Work out the finished part from the listing and answer in its coordinate system (mm). A direction names the side the tool comes from. Coordinates: 2 decimals unless noted, no trailing zeros. Write each loop counter-clockwise with the first axis right and the second up, starting at its lowest first coordinate (ties: lowest second). Pieces come first, ordered by that corner, then holes. Notation, with made-up numbers: (48.25, 21) - (106.25, 21) arc R21 ccw to (106.25, 48) - close; hole circle Ø4 at (-22, -15). An arc over 180 degrees is marked (long way). Use one line per item in the form item = value. Start each with the question number.
Item 1: Given pin 1 (4.5 mm diameter, centred on x = -11.5, z = 3.5, fed in from -Y); pin 2 (2.5 mm diameter, centred on y = 9, z = 4, fed in from +X); pin 3 (4.5 mm diameter, centred on x = -14.5, z = 2.5, fed in from +Y), each flat-ended and moving along its own axis, determine where each tip first touches the part or whether it passes through.
Item 2: A cutting plane is placed at C-C (y = 24.5). Write down the section's boundary in (x, z).
Item 3: A cutting plane is placed at B-B (z = 4.5). Write down the section's boundary in (x, y).
Item 4: Consider probe 1 along Y at (x, z) = (-14.5, 8); probe 2 along X at (y, z) = (24.75, 8.75); probe 3 along Y at (x, z) = (-24, 0.5). Determine where each line is inside the solid, lowest interval first.
Item 5: A cutting plane is placed at A-A (x = -13.25). Write down the section's boundary in (y, z).
Item 6: Determine the mould class of faces 1 (the cylindrical face through (-25.568, 29.715, 9.699)), 2 (the flat face through (-13, 15, 1)), 3 (the cylindrical face through (-19.606, 1.426, 5.056)) for opening direction Y: released by +Y, released by -Y, zero draft, split by the parting line, or undercut.
Item 7: For faces 4 (the cylindrical face through (-18.39, 9.58, 9.7)), 5 (the cylindrical face through (-13.68, 16.415, 9.699)), 6 (the flat face through (-18.103, 21, 5)), 7 (the flat face through (-18.103, 9, 5)), 8 (the cylindrical face through (-18.39, 20.91, 0.3)), determine the directions among +Z, -Z, +X, -X, +Y, -Y from which every point of the face is accessible in a straight line to the end or side of a thin tool.
from build123d import *

# Parameters (mm, degrees)
F0_W     = 15
F0_H     = 30
F1_DEPTH = 10
F2_W     = 3.4
F2_H     = 10
F2_W_2   = 1.4
F2_H_2   = 8
F3_DEPTH = 10
F4_R     = 5
F5_R     = 1
F6_R     = 0.99999


# Not quite as in the source:
# - a fillet or chamfer is up to 0.001 mm smaller than in the source, because OpenCascade refuses the exact size


with BuildPart() as f1:
    # F0 (on Top) → F1 (new body)
    with BuildSketch(Plane.XY):
        with Locations((-25.6027433276, 15)):
            Rectangle(F0_W, F0_H)
    extrude(amount=F1_DEPTH)

    # F2 (on face) → F3 (join)
    with BuildSketch(Plane.YZ.offset(-18.1027433276)):
        with Locations((15, 5)):
            Rectangle(F2_W, F2_H)
        with Locations((15, 5)):
            Rectangle(F2_W_2, F2_H_2, mode=Mode.SUBTRACT)
    extrude(amount=F3_DEPTH)

    # F4
    f4_edges = [f1.edges().sort_by_distance(p)[0] for p in [
        (-18.102743, 30, 5),
        (-33.102743, 30, 5),
        (-33.102743, 0, 5),
        (-18.102743, 0, 5),
    ]]
    fillet(f4_edges, radius=F4_R)

    # F5
    f5_edges = [f1.edges().sort_by_distance(p)[0] for p in [
        (-33.102743, 15, 10),
        (-31.638277, 28.535534, 10),
        (-25.602743, 30, 10),
        (-19.567209, 28.535534, 10),
        (-18.102743, 20.85, 10),
        (-18.102743, 9.15, 10),
        (-19.567209, 1.464466, 10),
        (-25.602743, 0, 10),
        (-31.638277, 1.464466, 10),
    ]]
    fillet(f5_edges, radius=F5_R)

    # F6 (radius 1 in the source; OpenCascade refuses exactly that, so slightly less here)
    f6_edges = [f1.edges().sort_by_distance(p)[0] for p in [
        (-18.102743, 20.85, 0),
        (-18.102743, 9.15, 0),
        (-19.567209, 1.464466, 0),
        (-25.602743, 0, 0),
        (-31.638277, 1.464466, 0),
        (-33.102743, 15, 0),
        (-31.638277, 28.535534, 0),
        (-25.602743, 30, 0),
        (-19.567209, 28.535534, 0),
        (-18.602743, 16.7, 10),
        (-13.102743, 16.7, 10),
        (-19.102743, 20.85, 10),
        (-8.102743, 15, 10),
        (-20.274316, 27.828427, 10),
        (-13.102743, 13.3, 10),
        (-25.602743, 29, 10),
        (-18.602743, 13.3, 10),
        (-30.93117, 27.828427, 10),
        (-19.102743, 9.15, 10),
        (-32.102743, 15, 10),
        (-20.274316, 2.171573, 10),
        (-30.93117, 2.171573, 10),
        (-25.602743, 1, 10),
    ]]
    fillet(f6_edges, radius=F6_R)


solid = f1.part
Answer:
q1.pin_1 = 13.3
q1.pin_2 = -18.1
q1.pin_3 = 16.7
q2.outline = (-33.1, 1) arc R1 ccw to (-32.1, 0) - (-19.1, 0) arc R1 ccw to (-18.1, 1) - (-18.1, 9) arc R1 ccw to (-19.1, 10) - (-32.1, 10) arc R1 ccw to (-33.1, 9) - close
q3.outline = (-33.1, 5) arc R5 ccw to (-28.1, 0) - (-23.1, 0) arc R5 ccw to (-18.1, 5) - (-18.1, 13.3) - (-8.1, 13.3) - (-8.1, 14.3) - (-18.1, 14.3) - (-18.1, 15.7) - (-8.1, 15.7) - (-8.1, 16.7) - (-18.1, 16.7) - (-18.1, 25) arc R5 ccw to (-23.1, 30) - (-28.1, 30) arc R5 ccw to (-33.1, 25) - close
q4.probe_1 = 13.3 to 14.3, 15.7 to 16.7
q4.probe_2 = -33.1 to -18.1
q4.probe_3 = 0.13 to 29.87
q5.outline = (13.3, 0) - (16.7, 0) - (16.7, 9) arc R1 ccw to (15.7, 10) - (14.3, 10) arc R1 ccw to (13.3, 9) - close; hole (14.3, 1) - (15.7, 1) - (15.7, 9) - (14.3, 9) - close
q6.face_1 = released by +Y
q6.face_2 = undercut
q6.face_3 = released by -Y
q7.face_4 = +Z, +X, -Y
q7.face_5 = +Z, +X, +Y
q7.face_6 = +Z, -Z, +X, +Y
q7.face_7 = +Z, -Z, +X, -Y
q7.face_8 = -Z, +X, +Y
